Can you work these out from the model? Positions are in its coordinate system, mm. A direction names the side the tool comes from. Round coordinates to 2 decimals unless told otherwise and drop trailing zeros. Loops run counter-clockwise (first coordinate to the right, second up) from the corner with the lowest first, then second, coordinate; pieces in that order, holes last.
```python
from build123d import *

# Parameters (mm, degrees)
SKETCH3_R           = 82.55
SKETCH3_R_2         = 19.05
BOSS_EXTRUDE2_DEPTH = 12.7
BOSS_EXTRUDE3_DEPTH = 3.175
CIRPATTERN1_COUNT   = 4
SKETCH8_R           = 8.686637198
CUT_EXTRUDE6_DEPTH  = 89.9


with BuildPart() as part:
    # Sketch3 → Boss-Extrude2 (new body)
    with BuildSketch(Plane(origin=(0, 0, 0), x_dir=(1, 0, 0), z_dir=(0, 1, 0))):
        Circle(SKETCH3_R)
        Circle(SKETCH3_R_2, mode=Mode.SUBTRACT)
    extrude(amount=BOSS_EXTRUDE2_DEPTH)

    # Sketch5 → Boss-Extrude3 (add, symmetric)
    with BuildSketch(Plane(origin=(0, 0, 0), x_dir=(0, 0, -1), z_dir=(1, 0, 0))):
        Polygon((-82.55, 88.9), (-44.45, 38.1), (-44.45, 12.7), (-95.25, 12.7), (-95.25, 88.9), align=None)
    boss_extrude3 = extrude(amount=BOSS_EXTRUDE3_DEPTH, both=True)

    # CirPattern1: Boss-Extrude3 ×4 about axis
    cirpattern1_axis = Axis((0, 0, 0), (0, 1, 0))
    for i in range(1, CIRPATTERN1_COUNT):
        add(boss_extrude3.rotate(cirpattern1_axis, i * 360 / CIRPATTERN1_COUNT))

    # Sketch8 → Cut-Extrude6 (cut, through all)
    with BuildSketch(Plane(origin=(0, 0, 0), x_dir=(1, 0, 0), z_dir=(0, 1, 0))):
        with Locations((43.68002845, -43.68002845)):
            Circle(SKETCH8_R)
        with Locations((-43.68002845, -43.68002845)):
            Circle(SKETCH8_R)
        with Locations((-43.68002845, 43.68002845)):
            Circle(SKETCH8_R)
        with Locations((43.68002845, 43.68002845)):
            Circle(SKETCH8_R)
    extrude(amount=CUT_EXTRUDE6_DEPTH, mode=Mode.SUBTRACT)


solid = part.part
```
(1) Suppose I cut it at B-B (y = 68.5). Write out the boundary of the cut face in (x, z) (3 decimals).
(2) We'd pull the mould along Z, two halves only. Please class faces 6 (the flat face through (0, 50, -95.25)), 7 (the flat face through (0, 63.9, 63.8)), 8 (the flat face through (75, 43, 3.175)), 9 (the flat face through (-95.25, 50, 0)): released by +Z, released by -Z, zero draft, split by the parting line, or undercut.
(3) Suppose I cut it at D-D (x = -68). Write out the boundary of the cut face in (y, z) (3 decimals).
(4) If I drill on line 1 (Z direction, x = 0, y = 6.75); line 2 (X direction, y = 36, z = -76) (3 decimals), over which ranges is the centre line in solid material (lowest first)?
(5) Which directions (+Z, -Z, +X, -X, +Y, -Y) give clear straight access to the entire face, cutting with the end or side of a thin tool? Please do faces 1 (the flat face through (-75, 43, -3.175)), 2 (the flat face through (-3.175, 43, 75)), 3 (the flat face through (-89, 12.7, 0)), 4 (the flat face through (3.175, 43, 75)), 5 (the flat face through (0, 12.7, -89)).
(6) Suppose I cut it at C-C (x = 0). Write out the boundary of the cut face in (y, z).
(7) For pin 1 (7 mm diameter, centred on x = 0, z = -91, fed in from -Y); pin 2 (3 mm diameter, centred on x = -55, y = 50, fed in from +Z) (3 decimals); pin 3 (22.5 mm diameter, centred on x = -43.68, z = -43.68, fed in from +Y), each with a flat end and sliding along its axis, tell me the tip position at first contact or that it passes through.
(8) Suppose I cut it at A-A (z = 0). Write out the boundary of the cut face in (x, y), then the cut area to 3 significant figures.
Check result:
1. outline: (-95.25, -3.175) - (-67.25, -3.175) - (-67.25, 3.175) - (-95.25, 3.175) - close; (-3.175, -95.25) - (3.175, -95.25) - (3.175, -67.25) - (-3.175, -67.25) - close; (-3.175, 67.25) - (3.175, 67.25) - (3.175, 95.25) - (-3.175, 95.25) - close; (67.25, -3.175) - (95.25, -3.175) - (95.25, 3.175) - (67.25, 3.175) - close
2. face 6: released by -Z
2. face 7: undercut
2. face 8: released by +Z
2. face 9: zero draft
3. outline: (0, -46.803) - (12.7, -46.803) - (12.7, -3.175) - (69.5, -3.175) - (69.5, 3.175) - (12.7, 3.175) - (12.7, 46.803) - (0, 46.803) - close
4. line 1: z = -82.55 to -19.05, 19.05 to 82.55
4. line 2: x = -3.175 to 3.175
5. face 1: -Z, +X, -X, +Y
5. face 2: +Z, -Z, -X, +Y
5. face 3: +Z, -Z, -X, -Y
5. face 4: +Z, -Z, +X, +Y
5. face 5: -Z, +X, -X, -Y
6. outline: (0, -82.55) - (12.7, -82.55) - (12.7, -95.25) - (88.9, -95.25) - (88.9, -82.55) - (38.1, -44.45) - (12.7, -44.45) - (12.7, -19.05) - (0, -19.05) - close; (0, 19.05) - (12.7, 19.05) - (12.7, 44.45) - (38.1, 44.45) - (88.9, 82.55) - (88.9, 95.25) - (12.7, 95.25) - (12.7, 82.55) - (0, 82.55) - close
7. pin 1: stops at y = 12.7
7. pin 2: stops at z = 3.175
7. pin 3: stops at y = 12.7
8. outline: (-95.25, 12.7) - (-82.55, 12.7) - (-82.55, 0) - (-19.05, 0) - (-19.05, 12.7) - (-44.45, 12.7) - (-44.45, 38.1) - (-82.55, 88.9) - (-95.25, 88.9) - close; (19.05, 0) - (82.55, 0) - (82.55, 12.7) - (95.25, 12.7) - (95.25, 88.9) - (82.55, 88.9) - (44.45, 38.1) - (44.45, 12.7) - (19.05, 12.7) - close
8. area: 7,420 mm2
